Autodesk Inventor part; units mm, degrees
ref_plane "YZ Plane" through (0, 0, 0) normal (1, 0, 0) x (0, 1, 0)
ref_plane "XZ Plane" through (0, 0, 0) normal (0, 1, 0) x (-1, 0, 0)
ref_plane "XY Plane" through (0, 0, 0) normal (0, 0, 1) x (1, 0, 0)
sketch "Эскиз1" plane through (0, 0, 0) normal (0, 0, 1) x (1, 0, 0)
  line L0 (-5, -82.5) -> (5, -82.5)
  line L1 (5, -82.5) -> (5, 82.5)
  line L2 (5, 82.5) -> (-5, 82.5)
  line L3 (-5, 82.5) -> (-5, -82.5)
  line L4 (-5, -82.5) -> (5, 82.5) construction
  line L5 (5, -82.5) -> (-5, 82.5) construction
  line L6 (-5, 82.5) -> (0, 82.5)
  line L7 (0, 82.5) -> (0, 77.5)
  line L8 (0, 77.5) -> (-5, 77.5)
  line L9 (-5, 77.5) -> (-5, 82.5)
  circle A0 centre (0, 77.5) radius 1.5
  line L10 (-5, 82.5) -> (5, 82.5)
  line L11 (5, 82.5) -> (5, 87.5)
  line L12 (5, 87.5) -> (-5, 87.5)
  line L13 (-5, 87.5) -> (-5, 82.5)
  circle A1 centre (0, 82.5) radius 1.5
  line L14 (-1.5, 82.5) -> (-1.5, 77.5)
  line L15 (1.5, 77.5) -> (1.5, 82.5)
  arc A2 (5, 82.5) -> (-5, 82.5) centre (0, 82.5) ccw
  line L16 (0, 77.5) -> (-5, 77.5)
  line L17 (-5, 77.5) -> (-5, 37.5)
  line L18 (-5, 37.5) -> (0, 37.5)
  line L19 (0, 37.5) -> (0, 77.5)
  circle A3 centre (0, 37.5) radius 1.5
  line L20 (-5, -82.5) -> (0, -82.5)
  line L21 (0, -82.5) -> (0, -77.5)
  line L22 (0, -77.5) -> (-5, -77.5)
  line L23 (-5, -77.5) -> (-5, -82.5)
  line L24 (-5, -82.5) -> (10, -82.5)
  line L25 (10, -82.5) -> (10, -72.5)
  line L26 (10, -72.5) -> (-5, -72.5)
  line L27 (-5, -72.5) -> (-5, -82.5)
  circle A4 centre (5, -77.5) radius 1.5
  point P0 (0, 0)
  point P1 (5, -72.5)
  dimension "d0" = 10
  dimension "d1" = 165
  dimension "d2" = 5
  dimension "d3" = 3
  dimension "d4" = 5
  dimension "d5" = 3
  dimension "d6" = 40
  dimension "d7" = 3
  dimension "d8" = 5
  dimension "d12" = 15
  dimension "d13" = 10
  dimension "d14" = 3
extrude "Выдавливание1" add sketch "Эскиз1" along normal blind 3 contours L3 L22 L21 L0 | L21 L22 L3 L26 L1 A4 L0 | L1 A4 L26 L25 L24 | L3 L18 A3 L19 A0 L15 L2 L1 L26 | L3 L8 A0 L19 A3 L18 | L3 L2 L14 L8 | L2 A1 A2
properties part number "пиналка_1"
The listing builds one solid part. Answer for the finished solid, in the listing's coordinates (mm). A direction names the side the tool comes from. Round coordinates to 2 decimals unless told otherwise and drop trailing zeros. Loops run counter-clockwise (first coordinate to the right, second up) from the corner with the lowest first, then second, coordinate; pieces in that order, holes last. Notation, with made-up numbers: M -0.5,-36.5 L 22.5,-36.5 A21 ccw 22.5,-31.5 Z; hole C 52.5,7 d1. An arc over 180 degrees is marked long. Return JSON: item names as keys, results as strings.
Q1. Each of these flat-tipped pins is pushed along its axis until it touches: pin 1 Ø1.5 at (x, z) = (1, 2) entering from +Y; pin 2 Ø3 at (x, y) = (4.5, -32.5) entering from -Z; pin 3 Ø0.9 at (x, z) = (7, 2) entering from +Y; pin 4 Ø2.5 at (x, y) = (5, -77.5) entering from +Z. Where does it stop, or does it pass through?
Results list:
{"pin 1": "stops at y = 87.49", "pin 2": "stops at z = 0", "pin 3": "stops at y = -72.5", "pin 4": "passes through"}
Q2. Which of the six approach directions +Z, -Z, +X, -X, +Y, -Y give full straight-line access (tool end or side, diameter ignored) to faces 4 (the face through (1.5, 80, 1)), 5 (the face through (5, 4, 1)), 6 (the face through (1, 4, 3))?
Results list:
{"face 4": "+Z, -Z", "face 5": "+Z, -Z, +X, +Y", "face 6": "+Z, +X, -X, +Y, -Y"}
Q3. Find the intervals of material crossed by line 1 along Y through (x, z) = (0, 1.95); line 2 along X through (y, z) = (-77.5, 1.9); line 3 along Y through (x, z) = (5.25, 0.5), in increasing order. Write a range as from..to.
Results list:
{"line 1": "y = -82.5..36, 39..76, 84..87.5", "line 2": "x = -5..3.5, 6.5..10", "line 3": "y = -82.5..-78.98, -76.02..-72.5"}
Q4. Find section B-B, the plane z = 0.55. Determine the outline of the cut face in (x, y).
Results list:
{"outline": "M -5,-82.5 L 10,-82.5 L 10,-72.5 L 5,-72.5 L 5,82.5 A5 ccw -5,82.5 Z; hole C 0,37.5 d3; hole M -1.5,77.5 A1.5 ccw 1.5,77.5 L 1.5,82.5 A1.5 ccw -1.5,82.5 Z; hole C 5,-77.5 d3"}
Q5. Find section C-C, the plane y = -77.5. Determine the outline of the cut face in (x, z), plus the area to 3 significant figures.
Results list:
{"outline": "M -5,0 L 3.5,0 L 3.5,3 L -5,3 Z; M 6.5,0 L 10,0 L 10,3 L 6.5,3 Z", "area": "36.0 mm2"}
Q6. The mould has two halves that part along Y. Classify faces 1 (the face through (-5, 1, 1)), 2 (the face through (0, 84, 1)), 3 (the face through (2, -82.5, 1)): released by +Y, released by -Y, zero draft, split by the parting line, or undercut.
Results list:
{"face 1": "zero draft", "face 2": "undercut", "face 3": "released by -Y"}
Q7. Find section A-A, the plane y = 37.5. Determine the outline of the cut face in (x, z).
Results list:
{"outline": "M -5,0 L -1.5,0 L -1.5,3 L -5,3 Z; M 1.5,0 L 5,0 L 5,3 L 1.5,3 Z"}
Q8. Find section D-D, the plane x = 8. Determine the outline of the cut face in (y, z), plus the area to 3 significant figures.
Results list:
{"outline": "M -82.5,0 L -72.5,0 L -72.5,3 L -82.5,3 Z", "area": "30.0 mm2"}
